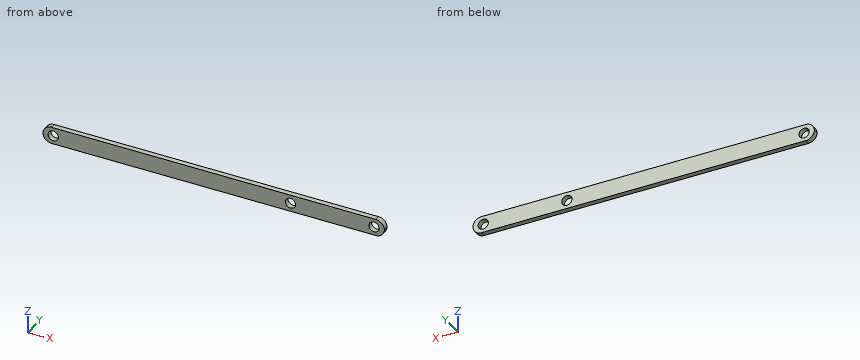
from build123d import *

# Parameters (mm, degrees)
SKETCH2_W           = 200
SKETCH2_H           = 10
BOSS_EXTRUDE1_DEPTH = 3
SKETCH3_R           = 3
CUT_EXTRUDE1_DEPTH  = 201.272314612
SKETCH4_R           = 3
CUT_EXTRUDE2_DEPTH  = 201.272314612
FILLET1_R           = 5
FILLET2_R           = 5
SKETCH5_R           = 3
CUT_EXTRUDE3_DEPTH  = 201.272314612


with BuildPart() as part:
    # Sketch2 → Boss-Extrude1 (new body)
    with BuildSketch(Plane(origin=(0, 0, 0), x_dir=(1, 0, 0), z_dir=(0, 1, 0))):
        with Locations((100, 5)):
            Rectangle(SKETCH2_W, SKETCH2_H)
    extrude(amount=BOSS_EXTRUDE1_DEPTH)

    # Sketch3 → Cut-Extrude1 (cut, through all)
    with BuildSketch(Plane(origin=(0, 3, 0), x_dir=(1, 0, 0), z_dir=(0, 1, 0))):
        with Locations(Location((6, 5, 0), (0, 0, 270))):
            Circle(SKETCH3_R)
    extrude(amount=-CUT_EXTRUDE1_DEPTH, mode=Mode.SUBTRACT)

    # Sketch4 → Cut-Extrude2 (cut, through all)
    with BuildSketch(Plane(origin=(0, 3, 0), x_dir=(1, 0, 0), z_dir=(0, 1, 0))):
        with Locations(Location((194, 5, 0), (0, 0, 270))):
            Circle(SKETCH4_R)
    extrude(amount=-CUT_EXTRUDE2_DEPTH, mode=Mode.SUBTRACT)

    # Fillet1
    fillet1_edges = [part.edges().sort_by_distance(p)[0] for p in [
        (0, 1.5, -10),
        (0, 1.5, 0),
    ]]
    fillet(fillet1_edges, radius=FILLET1_R - 0.0001)  # a hair under: the kernel refuses the full size

    # Fillet2
    fillet2_edges = [part.edges().sort_by_distance(p)[0] for p in [
        (200, 1.5, -10),
        (200, 1.5, 0),
    ]]
    fillet(fillet2_edges, radius=FILLET2_R - 0.0001)  # a hair under: the kernel refuses the full size

    # Sketch5 → Cut-Extrude3 (cut, through all)
    with BuildSketch(Plane(origin=(0, 3, 0), x_dir=(1, 0, 0), z_dir=(0, 1, 0))):
        with Locations(Location((145, 5, 0), (0, 0, 270))):
            Circle(SKETCH5_R)
    extrude(amount=-CUT_EXTRUDE3_DEPTH, mode=Mode.SUBTRACT)


solid = part.part
Input: part model. Units: mm. Frame: model coordinates. Coordinates: 2 decimals unless noted, no trailing zeros. Loops run counter-clockwise (first coordinate to the right, second up) from the corner with the lowest first, then second, coordinate; pieces in that order, holes last. Notation, with made-up numbers: (72, 52.25) -> (103, 52.25) arc R17 ccw to (103, 60.25) -> close; hole circle Ø10 at (28.5, -38.75). An arc over 180 degrees is marked (long way). Write each question's results on one line, items separated by ' | '. Start each with the question number.
Q1. Section B-B, the plane y = 0.9. State how many separate pieces and enclosed holes the cut face has, plus the area to 3 significant figures.
Q2. Section A-A, the plane x = 145. Return the cut outline in (y, z).
Q3. Ray query, line 1 (X direction, y = 1.8, z = -5); line 2 (X direction, y = 2.3, z = -2.25). Return the intervals inside material, ascending. Write a range as from..to.
Found:
1) separate pieces: 1 | enclosed holes: 3 | area: 1,890 mm2
2) outline: (0, -10) -> (3, -10) -> (3, -8) -> (0, -8) -> close; (0, -2) -> (3, -2) -> (3, 0) -> (0, 0) -> close
3) line 1: 0..3, 9..142, 148..191, 197..200 | line 2: 0.82..4.8, 7.2..143.8, 146.2..192.8, 195.2..199.18
